Here's how the part is built. I have some questions about the finished solid (model axes, mm). A direction names the side the tool comes from. Give positions to 0.01 mm unless a question says otherwise; leave off trailing zeros. Write each loop counter-clockwise with the first axis right and the second up, starting at its lowest first coordinate (ties: lowest second). Pieces come first, ordered by that corner, then holes. Notation, with made-up numbers: (30, 23) -> (47, 23) arc R13 ccw to (47, 30) -> close; hole circle Ø4 at (66, 24.25). An arc over 180 degrees is marked (long way). Put each result on its own line as item: value. Start each with the question number.
from build123d import *

# Parameters (mm, degrees)
SKETCH1_W           = 100
SKETCH1_H           = 110
SKETCH1_R           = 2.5
SKETCH1_R_2         = 1.5
BOSS_EXTRUDE1_DEPTH = 3


with BuildPart() as part:
    # Sketch1 → Boss-Extrude1 (new body)
    with BuildSketch(Plane.XY):
        Rectangle(SKETCH1_W, SKETCH1_H)
        with Locations((-25, -45)):
            Circle(SKETCH1_R, mode=Mode.SUBTRACT)
        with Locations((25, -45)):
            Circle(SKETCH1_R, mode=Mode.SUBTRACT)
        with Locations((-15.5, 24.997203367)):
            Circle(SKETCH1_R_2, mode=Mode.SUBTRACT)
        with Locations((-7.752421955, 38.421995442)):
            Circle(SKETCH1_R_2, mode=Mode.SUBTRACT)
        with Locations((7.747578045, 38.424792075)):
            Circle(SKETCH1_R_2, mode=Mode.SUBTRACT)
        with Locations((15.5, 25.002796633)):
            Circle(SKETCH1_R_2, mode=Mode.SUBTRACT)
        with Locations((7.752421955, 11.578004558)):
            Circle(SKETCH1_R_2, mode=Mode.SUBTRACT)
        with Locations((-7.747578045, 11.575207925)):
            Circle(SKETCH1_R_2, mode=Mode.SUBTRACT)
        with BuildLine():
            Line((5.910876507, 33.185052569), (5.959490464, 19.526769566))
            ThreePointArc((5.959490464, 19.526769566), (0.010605831, 13.546039163), (-5.959528213, 19.505557938))
            Line((-5.959528213, 19.505557938), (-5.959528213, 33.944996934))
            ThreePointArc((-5.959528213, 33.944996934), (0.380750058, 39.892349783), (5.910876507, 33.185052569))
        make_face(mode=Mode.SUBTRACT)
    extrude(amount=BOSS_EXTRUDE1_DEPTH)


solid = part.part
1) Which directions (+Z, -Z, +X, -X, +Y, -Y) give clear straight access to the entire face, cutting with the end or side of a thin tool? Please do faces 5 (the flat face through (-50, -1, 1)), 6 (the cylindrical face through (0.142, 13.548, 1.479)).
2) I want a section at D-D, the plane z = 0.55. State how many separate pieces and enclosed holes the cut face has, and give its area (3 significant figures).
3) Thinking about a two-plate mould opening in Y: for faces 1 (the flat face through (-1, 1, 3)), 2 (the flat face through (-1, -55, 1)), 3 (the flat face through (-1, 55, 1)), 4 (the cylindrical face through (6.254, 11.644, 1.479)), which applies, released by +Y, released by -Y, zero draft, split by the parting line, or undercut?
4) I need wall thicknesses on probe 1 along Y at (x, z) = (7.5, 0.4); probe 2 along X at (y, z) = (19, 2.9); probe 3 along Y at (x, z) = (-9, 0.3). Which ranges of each line are inside material? Lowest first, please.
5) I want a section at B-B, the plane y = -45. Write out the boundary of the cut face in (x, z).
6) I want a section at A-A, the plane x = 0. Write out the boundary of the cut face in (y, z).
7) I want a section at C-C, the plane x = 25. Write out the boundary of the cut face in (y, z), and give its area (3 significant figures).
Established:
1. face 5: +Z, -Z, -X, +Y, -Y
1. face 6: +Z, -Z
2. separate pieces: 1
2. enclosed holes: 9
2. area: 10,600 mm2
3. face 1: zero draft
3. face 2: released by -Y
3. face 3: released by +Y
3. face 4: undercut
4. probe 1: y = -55 to 10.1, 13.06 to 36.95, 39.9 to 55
4. probe 2: x = -50 to -5.94, 5.94 to 50
4. probe 3: y = -55 to 10.75, 12.4 to 37.59, 39.25 to 55
5. outline: (-50, 0) -> (-27.5, 0) -> (-27.5, 3) -> (-50, 3) -> close; (-22.5, 0) -> (22.5, 0) -> (22.5, 3) -> (-22.5, 3) -> close; (27.5, 0) -> (50, 0) -> (50, 3) -> (27.5, 3) -> close
6. outline: (-55, 0) -> (13.55, 0) -> (13.55, 3) -> (-55, 3) -> close; (39.9, 0) -> (55, 0) -> (55, 3) -> (39.9, 3) -> close
7. outline: (-55, 0) -> (-47.5, 0) -> (-47.5, 3) -> (-55, 3) -> close; (-42.5, 0) -> (55, 0) -> (55, 3) -> (-42.5, 3) -> close
7. area: 315 mm2
